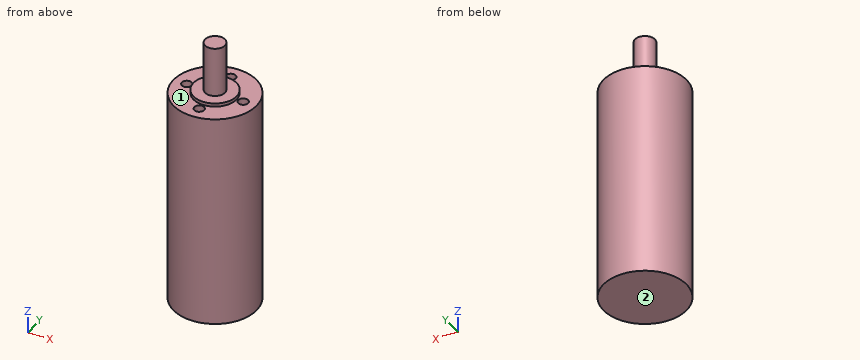
```python
from build123d import *

# Parameters (mm, degrees)
ESBO_O1_R                = 12.5
RESSALTO_EXTRUS_O1_DEPTH = 65
ESBO_O2_R                = 6.5
RESSALTO_EXTRUS_O2_DEPTH = 1
ESBO_O3_R                = 3
RESSALTO_EXTRUS_O3_DEPTH = 15
ESBO_O4_R                = 1.5
CORTE_EXTRUS_O1_DEPTH    = 4
PADR_OCIRCULAR1_COUNT    = 4


with BuildPart() as part:
    # Esboço1 → Ressalto-extrusão1 (new body)
    with BuildSketch(Plane.XY):
        Circle(ESBO_O1_R)
    extrude(amount=RESSALTO_EXTRUS_O1_DEPTH)

    # Esboço2 → Ressalto-extrusão2 (add)
    with BuildSketch(Plane.XY.offset(65)):
        Circle(ESBO_O2_R)
    extrude(amount=RESSALTO_EXTRUS_O2_DEPTH)

    # Esboço3 → Ressalto-extrusão3 (add)
    with BuildSketch(Plane.XY.offset(66)):
        Circle(ESBO_O3_R)
    extrude(amount=RESSALTO_EXTRUS_O3_DEPTH)

    # Esboço4 → Corte-extrusão1 (cut)
    with BuildSketch(Plane.XY.offset(65)):
        with Locations((0, -8.5)):
            Circle(ESBO_O4_R)
    corte_extrus_o1 = extrude(amount=-CORTE_EXTRUS_O1_DEPTH, mode=Mode.SUBTRACT)

    # PadrãoCircular1: Corte-extrusão1 ×4 about axis
    padr_ocircular1_axis = Axis((0, 0, 0), (0, 0, 1))
    for i in range(1, PADR_OCIRCULAR1_COUNT):
        add(corte_extrus_o1.rotate(padr_ocircular1_axis, i * 360 / PADR_OCIRCULAR1_COUNT), mode=Mode.SUBTRACT)


solid = part.part
```
The listing builds one solid part. Answer for the finished solid, in the listing's coordinates (mm). Face numbers are marked on the shaded views. A direction names the side the tool comes from. Give positions to 0.01 mm unless a question says otherwise; leave off trailing zeros. Order: outer loops, then holes, each group sorted by start corner. A loop starts at its lowest first (then second) coordinate and runs counter-clockwise, first axis right, second up. Notation, with made-up numbers: (-23.5, 9) -> (-10.5, 9) arc R29 ccw to (-10.5, 35) -> close; hole circle Ø8 at (68, 10). An arc over 180 degrees is marked (long way). One line per item, written item: value.
1) Find section C-C, the plane z = 27. Determine the outline of the cut face in (x, y).
Reported:
outline: circle Ø25 at (0, 0)
2) Find section A-A, the plane y = 0. Determine the outline of the cut face in (x, z).
Reported:
outline: (-12.5, 0) -> (12.5, 0) -> (12.5, 65) -> (10, 65) -> (10, 61) -> (7, 61) -> (7, 65) -> (6.5, 65) -> (6.5, 66) -> (3, 66) -> (3, 81) -> (-3, 81) -> (-3, 66) -> (-6.5, 66) -> (-6.5, 65) -> (-7, 65) -> (-7, 61) -> (-10, 61) -> (-10, 65) -> (-12.5, 65) -> close
3) Find section D-D, the plane y = -7.75. Determine the outline of the cut face in (x, z), plus the area to 3 significant figures.
Reported:
outline: (-9.81, 0) -> (9.81, 0) -> (9.81, 65) -> (1.3, 65) -> (1.3, 61) -> (-1.3, 61) -> (-1.3, 65) -> (-9.81, 65) -> close
area: 1,260 mm^2
4) A tool of negligible diameter and unlimited length cuts with its end or side. For the marked faces 1 and 2, from which of +Z, -Z, +X, -X, +Y, -Y can it reach the whole face along a straight path? Write none if from no direction.
Reported:
face 1: +Z
face 2: -Z, +X, -X, +Y, -Y
5) Find the intervals of material crossed by line 1 (Y direction, x = 0, z = 61.95); line 2 (Z direction, x = -9, y = -1.75); line 3 (X direction, y = 8.5, z = 64.05), in increasing order.
Reported:
line 1: y = -12.5 to -10, -7 to 7, 10 to 12.5
line 2: z = 0 to 65
line 3: x = -9.17 to -1.5, 1.5 to 9.17
6) Flat-ended cylindrical pins translate along their axes: P1, Ø0.9, axis at x = -0.5, y = 8, coming from the +Z side; P2, Ø5, axis at x = 8.5, y = 0, coming from the -Z side; P3, Ø12, axis at x = 7, z = 35.5, coming from the -Y side; P4, Ø2.5, axis at x = -8, y = 0, coming from the +Z side. Find the tip coordinate at first contact, or state that the pin passes through.
Reported:
P1: stops at z = 61
P2: stops at z = 0
P3: stops at y = -12.46
P4: stops at z = 65
7) Find section B-B, the plane x = -8.5. Determine the outline of the cut face in (y, z), plus the area to 3 significant figures.
Reported:
outline: (-9.17, 0) -> (9.17, 0) -> (9.17, 65) -> (1.5, 65) -> (1.5, 61) -> (-1.5, 61) -> (-1.5, 65) -> (-9.17, 65) -> close
area: 1,180 mm^2
